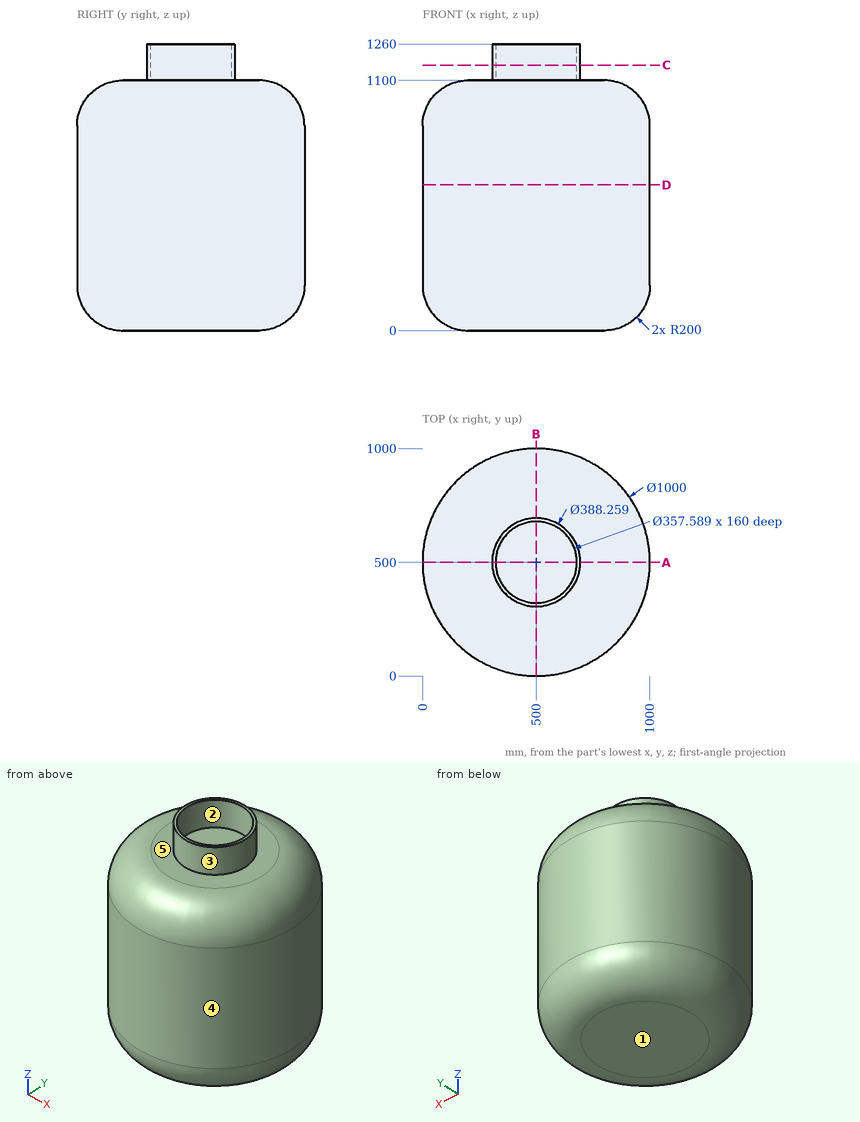
Answer from the drawing. Dimensions are ordinates in mm from the lowest x, y and z of the part. A direction names the side the tool comes from. Coordinates: 2 decimals unless noted, no trailing zeros. Write each loop counter-clockwise with the first axis right and the second up, starting at its lowest first coordinate (ties: lowest second). Pieces come first, ordered by that corner, then holes. Notation, with made-up numbers: M -17,2.25 L 32,2.25 A22 cw 32,9.25 Z; hole C 78,-18 d1. An arc over 180 degrees is marked long. Use a Markdown table: item, result.
Q1. The part is cut by section C-C, the plane z = 1167. Write down the section's boundary in (x, y) (1 decimal), then the cut area to 3 significant figures.
Answer block:
| item | result |
|---|---|
| outline | C 500,500 d388.3; hole C 500,500 d357.6 |
| area | 18,000 mm2 |
Q2. Which of the six approach directions +Z, -Z, +X, -X, +Y, -Y give full straight-line access (tool end or side, diameter ignored) to the marked faces 4 and 5?
Answer block:
| item | result |
|---|---|
| face 4 | +Z, -Z |
| face 5 | +Z |
Q3. Determine the mould class of the marked faces 1, 2 and 3 for opening direction Y: released by +Y, released by -Y, zero draft, split by the parting line, or undercut.
Answer block:
| item | result |
|---|---|
| face 1 | zero draft |
| face 2 | undercut |
| face 3 | split by the parting line |
Q4. The part is cut by section D-D, the plane z = 640.5. Write down the section's boundary in (x, y).
Answer block:
| item | result |
|---|---|
| outline | C 500,500 d1000 |
Q5. Straight lines are drawn through the part: L1, parallel to Y at x = 500, z = 1218.5 (1 decimal); L2, parallel to Z at x = 481, y = 705; L3, parallel to Y at x = 807, z = 398 (1 decimal). For each, find the intervals that lie inside material, in ascending order. Write a range as [from, to].
Answer block:
| item | result |
|---|---|
| L1 | y = [305.9, 321.2], [678.8, 694.1] |
| L2 | z = [0, 1100] |
| L3 | y = [105.3, 894.7] |
Q6. Each of these flat-tipped pins is pushed along its axis until it touches: pin 1 Ø12 at (y, z) = (199.5, 614) entering from -X; pin 2 Ø3 at (x, z) = (710.5, 1044) entering from +Y; pin 3 Ø12 at (x, z) = (438, 343) entering from -Y. Where does it stop, or does it pass through?
Answer block:
| item | result |
|---|---|
| pin 1 | stops at x = 95.93 |
| pin 2 | stops at y = 886.94 |
| pin 3 | stops at y = 3.15 |
Q7. The part is cut by section A-A, the plane y = 500. Write down the section's boundary in (x, z) (1 decimal), then the cut area to 3 significant figures.
Answer block:
| item | result |
|---|---|
| outline | M 0,200 A200 ccw 200,0 L 800,0 A200 ccw 1000,200 L 1000,900 A200 ccw 800,1100 L 694.1,1100 L 694.1,1260 L 678.8,1260 L 678.8,1100 L 321.2,1100 L 321.2,1260 L 305.9,1260 L 305.9,1100 L 200,1100 A200 ccw 0,900 Z |
| area | 1,070,000 mm2 |
